Model file for the job. Use its own axes, mm. Round coordinates to 2 decimals unless told otherwise and drop trailing zeros. Loops run counter-clockwise (first coordinate to the right, second up) from the corner with the lowest first, then second, coordinate; pieces in that order, holes last. Notation, with made-up numbers: (13, 9) -> (40, 9) arc R31 cw to (40, 37) -> close; hole circle Ø6 at (75, 48.5). An arc over 180 degrees is marked (long way). Use a Markdown table: item, result.
from build123d import *

# Parameters (mm, degrees)
F1_DEPTH = 25.4
F2_R     = 5.08
F3_R     = 5.08


with BuildPart() as f1:
    # F0 (on Top) → F1 (new body)
    with BuildSketch(Plane.XY):
        with BuildLine():
            Line((31.895727, 5.925444), (31.895727, 20.89718))
            Line((31.895727, 20.89718), (-25.545727, 20.89718))
            ThreePointArc((-25.545727, 20.89718), (-30.035855, 19.037308), (-31.895727, 14.54718))
            Line((-31.895727, 14.54718), (-31.895727, -14.54718))
            ThreePointArc((-31.895727, -14.54718), (-30.035855, -19.037308), (-25.545727, -20.89718))
            Line((-25.545727, -20.89718), (5.073103, -20.89718))
            ThreePointArc((5.073103, -20.89718), (24.039562, -13.041015), (31.895727, 5.925444))
        make_face()
    extrude(amount=F1_DEPTH)

    # F2
    f2_edges = [f1.edges().sort_by_distance(p)[0] for p in [
        (24.039562, -13.041015, 25.4),
        (31.895727, 13.411312, 25.4),
        (3.175, 20.89718, 25.4),
        (-30.035855, 19.037308, 25.4),
        (-31.895727, 0, 25.4),
        (-10.236312, -20.89718, 25.4),
        (-30.035855, -19.037308, 25.4),
    ]]
    fillet(f2_edges, radius=F2_R)

    # F3
    f3_edges = [f1.edges().sort_by_distance(p)[0] for p in [
        (3.175, 20.89718, 0),
        (31.895727, 13.411312, 0),
        (24.039562, -13.041015, 0),
        (-10.236312, -20.89718, 0),
        (-30.035855, -19.037308, 0),
        (-31.895727, 0, 0),
        (-30.035855, 19.037308, 0),
    ]]
    fillet(f3_edges, radius=F3_R)


solid = f1.part
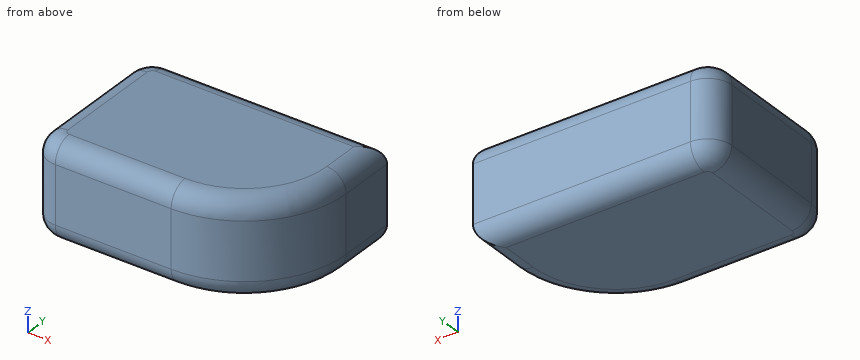
Q1. Flat gauge pins, fed straight in: pin 1 (1 mm diameter, centred on x = 8.5, y = -16.5, fed in from -Z); pin 2 (10 mm diameter, centred on y = -2, z = 12, fed in from +X); pin 3 (12 mm diameter, centred on y = 1, z = 8, fed in from +X). Where does each tip first touch, or does it go through?
Results list:
| item | result |
|---|---|
| pin 1 | stops at z = 0.02 |
| pin 2 | stops at x = 31.74 |
| pin 3 | stops at x = 31.9 |
Q2. Band-saw the part on A-A, the plane z = 8.5. Give the cut face in (x, y), plus the area to 3 significant figures.
Results list:
| item | result |
|---|---|
| outline | (-31.9, -14.55) arc R6.35 ccw to (-25.55, -20.9) -> (5.07, -20.9) arc R26.82 ccw to (31.9, 5.93) -> (31.9, 20.9) -> (-25.55, 20.9) arc R6.35 ccw to (-31.9, 14.55) -> close |
| area | 2,490 mm² |
Q3. Band-saw the part on B-B, the plane x = -3. Give the cut face in (y, z).
Results list:
| item | result |
|---|---|
| outline | (-20.9, 5.08) arc R5.08 ccw to (-15.82, 0) -> (15.82, 0) arc R5.08 ccw to (20.9, 5.08) -> (20.9, 20.32) arc R5.08 ccw to (15.82, 25.4) -> (-15.82, 25.4) arc R5.08 ccw to (-20.9, 20.32) -> close |
Q4. Drill centre lines: L1, parallel to Z at x = 18, y = 16; L2, parallel to Y at x = -11, z = 20.5; L3, parallel to X at y = -7, z = 17.25. Where is each one in solid material? Low to high. Write a range as from..to.
Results list:
| item | result |
|---|---|
| L1 | z = 0..25.4 |
| L2 | y = -20.89..20.89 |
| L3 | x = -31.9..28.58 |
